Check sheet for the modelled part. Datum: model origin and axes. Units: mm. A direction names the side the tool comes from. Coordinates: 2 decimals unless noted, no trailing zeros. Order: outer loops, then holes, each group sorted by start corner. A loop starts at its lowest first (then second) coordinate and runs counter-clockwise, first axis right, second up.
from build123d import *

# Parameters (mm, degrees)
F1_DEPTH = 5
F3_DEPTH = 5
F4_W     = 5
F4_H     = 5.42134
F5_DEPTH = 5


with BuildPart() as f1:
    # F0 (on Top) → F1 (new body)
    with BuildSketch(Plane.XY):
        Polygon((28, -8.65), (28, 8.65), (-28, 8.65), (-28, -8.65), (-28, -13.65), (28, -13.65), align=None)
    extrude(amount=F1_DEPTH)

    # F2 (on face) → F3 (cut)
    with BuildSketch(Plane.XY.offset(5)):
        with BuildLine():
            ThreePointArc((-18.559123, 4.10952), (-18.514825, 4.378148), (-18.5, 4.65))
            ThreePointArc((-18.5, 4.65), (-23.485175, 4.921852), (-18.559123, 4.10952))
        make_face()
        with BuildLine():
            ThreePointArc((23.5, 4.65), (20.728148, 7.135175), (18.559123, 4.10952))
            ThreePointArc((18.559123, 4.10952), (21.271852, 2.164825), (23.5, 4.65))
        make_face()
    extrude(amount=-F3_DEPTH, mode=Mode.SUBTRACT)

    # F4 (on face) → F5 (cut)
    with BuildSketch(Plane.XY.offset(5)):
        with Locations((-15, -10.93933)):
            Rectangle(F4_W, F4_H)
        with Locations((14.643573, -10.93933)):
            Rectangle(F4_W, F4_H)
    extrude(amount=-F5_DEPTH, mode=Mode.SUBTRACT)


solid = f1.part
(1) Cross-section at B-B (x = -21). Enter the section's corners in (y, z).
Filled in:
outline: (-13.65, 0) - (2.15, 0) - (2.15, 5) - (-13.65, 5) - close; (7.15, 0) - (8.65, 0) - (8.65, 5) - (7.15, 5) - close
(2) Tool access check on faces 4 (the flat face through (-17.5, -11, 3)), 5 (the flat face through (22, -13.65, 2)). Record the directions out of +Z, -Z, +X, -X, +Y, -Y that give a thin tool (end or side, any length) a straight path to the whole face; none if there is none.
Filled in:
face 4: +Z, -Z, -Y
face 5: +Z, -Z, +X, -X, -Y
(3) Cross-section at C-C (x = 21.5). Enter the section's corners in (y, z).
Filled in:
outline: (-13.65, 0) - (2.2, 0) - (2.2, 5) - (-13.65, 5) - close; (7.1, 0) - (8.65, 0) - (8.65, 5) - (7.1, 5) - close
(4) Release check for a two-part mould opening along X. For faces 1 (the flat face through (0, 8.65, 2)), 2 (the flat face through (28, -3, 2)), 3 (the flat face through (12.144, -11, 3)) record: +X half, -X half, draft (parallel to the pull), parting line (faces both ways), or undercut.
Filled in:
face 1: draft
face 2: +X half
face 3: undercut
(5) Thickness scan on probe 1 along X at (y, z) = (4.65, 1.8); probe 2 along X at (y, z) = (-12.25, 2.05); probe 3 along Y at (x, z) = (21, 3.7). Record the ranges inside material, lowest first.
Filled in:
probe 1: x = -28 to -23.5, -18.5 to 18.5, 23.5 to 28
probe 2: x = -28 to -17.5, -12.5 to 12.14, 17.14 to 28
probe 3: y = -13.65 to 2.15, 7.15 to 8.65
(6) Cross-section at A-A (z = 3.7). Enter the section's corners in (x, y), and give its area (3 significant figures).
Filled in:
outline: (-28, -13.65) - (-17.5, -13.65) - (-17.5, -8.23) - (-12.5, -8.23) - (-12.5, -13.65) - (12.14, -13.65) - (12.14, -8.23) - (17.14, -8.23) - (17.14, -13.65) - (28, -13.65) - (28, 8.65) - (-28, 8.65) - close; hole (-18.56, 4.11) arc R2.5 ccw to (-18.5, 4.65) arc R2.5 ccw (long way) to start; hole circle Ø5 at (21, 4.65)
area: 1,160 mm2
